from build123d import *

# Parameters (mm, degrees)
SOCKET_SKETCH_W = 16.2
SOCKET_SKETCH_H = 3.175


with BuildPart() as part:
    # Conn_T4_ORB8 Sketch → Conn_T4_ORB8 (revolve)
    with BuildSketch(Plane.XY, mode=Mode.PRIVATE) as conn_t4_orb8_sk:
        Polygon((13.3, 0), (13.3, 8.73), (0, 8.73), (0, 11.988), (-24.3, 11.988), (-24.3, 0), align=None)
    revolve(conn_t4_orb8_sk.sketch.rotate(Axis((-1000, 0, 0), (1, 0, 0)), 90), axis=Axis((-1000, 0, 0), (1, 0, 0)))

    # Socket Sketch → Socket (revolve, cut)
    with BuildSketch(Plane.XY, mode=Mode.PRIVATE) as socket_sk:
        with Locations((-17.2, 1.5875)):
            Rectangle(SOCKET_SKETCH_W, SOCKET_SKETCH_H)
    revolve(socket_sk.sketch.rotate(Axis((-1000, 0, 0), (1, 0, 0)), 90), axis=Axis((-1000, 0, 0), (1, 0, 0)), mode=Mode.SUBTRACT)


solid = part.part
The model under review builds one solid part; all positions refer to its coordinate system, in mm. A direction names the side the tool comes from. Round coordinates to 2 decimals unless told otherwise and drop trailing zeros. Order: outer loops, then holes, each group sorted by start corner. A loop starts at its lowest first (then second) coordinate and runs counter-clockwise, first axis right, second up. Notation, with made-up numbers: (-37.75, -7) - (-32.75, -7) arc R23 ccw to (-32.75, 22) - close; hole circle Ø11 at (46, 35.25). An arc over 180 degrees is marked (long way). Use one line per item in the form item = value.
Q1. Mouldability with a two-part tool opening along Z and no side actions: class faces 4 (the cylindrical face through (-12.32, -3.601, 11.434)), 5 (the flat face through (-9.1, 0, 0)), 6 (the flat face through (0, 9, -1)) as pulls with the +Z half, pulls with the -Z half, needs draft (parallel to the pull), parting line crosses it, or undercut.
Response values:
face_4 = parting line crosses it
face_5 = undercut
face_6 = needs draft
Q2. Clearance check with flat-ended pins moving along their axes: P1, Ø7.5, axis at y = 0, z = 0, coming from the -X side; P2, Ø3, axis at x = -6.5, z = 8.5, coming from the +Y side; P3, Ø6, axis at x = 7, z = 9, coming from the +Y side; P4, Ø1.9, axis at y = 0, z = 1.5, coming from the -X side. State where each tip first meets the part, or that it passes through.
Response values:
P1 = -24.3
P2 = 9.73
P3 = 6.34
P4 = -9.1
Q3. Add section A-A on y = 0. Give the boundary of the cut face in (x, z) (3 decimals).
Response values:
outline = (-24.3, -11.988) - (0, -11.988) - (0, -8.73) - (13.3, -8.73) - (13.3, 8.73) - (0, 8.73) - (0, 11.988) - (-24.3, 11.988) - (-24.3, 3.175) - (-9.1, 3.175) - (-9.1, -3.175) - (-24.3, -3.175) - close
Q4. Add section D-D on x = -17.5. Give the boundary of the cut face in (y, z) (3 decimals).
Response values:
outline = circle Ø23.976 at (0, 0); hole circle Ø6.35 at (0, 0)
Q5. To check wall thickness, follow line 1 (Y direction, x = -20.25, z = 0) (3 decimals); line 2 (X direction, y = -3.75, z = 9.25); line 3 (Y direction, x = -10.5, z = 2.25). State the ranges of each line that lie inside material, in increasing order.
Response values:
line_1 = -11.988 to -3.175, 3.175 to 11.988
line_2 = -24.3 to 0
line_3 = -11.77 to -2.24, 2.24 to 11.77
Q6. Tool access review of faces 1 (the cylindrical face through (-16.59, 1.93, -2.52)), 2 (the cylindrical face through (6.557, -8.656, -1.136)), 3 (the flat face through (13.3, 0, 0)): name each direction out of +Z, -Z, +X, -X, +Y, -Y from which nothing blocks a thin tool from reaching the whole face with its end or side.
Response values:
face_1 = -X
face_2 = +X
face_3 = +Z, -Z, +X, +Y, -Y
Q7. Add section C-C on x = -7. Give the boundary of the cut face in (y, z).
Response values:
outline = circle Ø23.98 at (0, 0)
